Work out the finished part from the listing and answer in its coordinate system (mm). Face numbers are marked on the shaded views. A direction names the side the tool comes from. Coordinates: 2 decimals unless noted, no trailing zeros. Order: outer loops, then holes, each group sorted by start corner. A loop starts at its lowest first (then second) coordinate and runs counter-clockwise, first axis right, second up. Notation, with made-up numbers: M -37,73 L -14,73 A33 cw -14,111 Z; hole C -18.5,85 d11. An arc over 180 degrees is marked long. Use a Markdown table: item, result.
Autodesk Inventor part; units mm, degrees
ref_plane "Work Plane3" through (44.45, 0, 0) normal (-0.342, 0.9397, 0) x (0, 0, -1)
ref_plane "YZ Plane" through (0, 0, 0) normal (1, 0, 0) x (0, 1, 0)
ref_plane "XZ Plane" through (0, 0, 0) normal (0, 1, 0) x (-1, 0, 0)
sketch "Sketch1" plane through (0, 0, 0) normal (0, 1, 0) x (-1, 0, 0)
  line L0 (0, 0) -> (-44.45, 0)
  line L1 (-44.45, 0) -> (-44.45, -25.4)
  line L2 (-44.45, -25.4) -> (0, -25.4)
  line L3 (0, -25.4) -> (0, 0)
  line L4 (-41.275, -25.4) -> (-41.275, 0)
  line L5 (-41.275, -19.05) -> (-44.45, -20.8831)
  line L6 (0, -12.7) -> (-44.45, -12.7) construction
  line L7 (-41.275, -6.35) -> (-44.45, -4.5169)
  point P0 (-44.45, -4.5169)
  point P1 (-41.275, -6.35)
  dimension "d0" = 44.45
  dimension "d7" = 25.4
  dimension "d10" = 3.175
  dimension "d11" = 12.7
  dimension "d12" = 60
extrude "Extrusion1" add sketch "Sketch1" along normal blind 19.05
sketch "Sketch3" plane through (0, 0, 0) normal (0, 0, 1) x (1, 0, 0)
  line L0 (0, 0) -> (44.45, 0)
  line L1 (44.45, 0) -> (44.45, 19.05)
  line L2 (0, 19.05) -> (44.45, 19.05)
  line L3 (0, 0) -> (0, 19.05)
  line L4 (24.8164, 19.05) -> (31.75, 0)
  dimension "d14" = 70
  dimension "d15" = 31.75
sweep "Sweep1" cut profiles "Sketch1" path "Sketch3" path curves L4 contours L4 L7 L1 L0 | L2 L1 L5 L4
ref_plane "Work Plane3" through (44.45, 0, 0) normal (-0.342, 0.9397, 0) x (0, 0, -1)
ref_plane "Work Plane2" through (44.45, 0, 0) normal (-0.9397, -0.342, 0) x (0, 0, -1)
sketch "Sketch5" plane through (44.45, 0, 0) normal (-0.342, 0.9397, 0) x (0, 0, -1)
  point P0 (12.7, 0)
hole "Hole2" at (44.45, 0, -12.7) direction (-0.342, 0.9397, 0) diameter 4.9784 end through all
split "Split1" plane through (44.45, 0, 0) removes the side toward (0.9397, 0.342, 0)
sketch "Sketch4" plane through (0, 19.05, 0) normal (0, 1, 0) x (1, 0, 0)
  line L0 (0, 0) -> (34.3414, 0) construction
  line L1 (0, 25.4) -> (0, 0) construction
  point P0 (17.1707, 12.7)
  point P1 (0, 12.7)
  point P2 (17.1707, 0)
hole "Hole1" at (17.1707, 19.05, -12.7) direction (0, -1, 0) diameter 10.0838 end through all counterbore diameter 15.875 counterbore depth 9.525
equation "\"d14\" = slopeAngle"
equation "\"d18\" = slopeAngle"
equation "\"slopeAngle\" = 70deg"
properties material "Steel, Alloy"
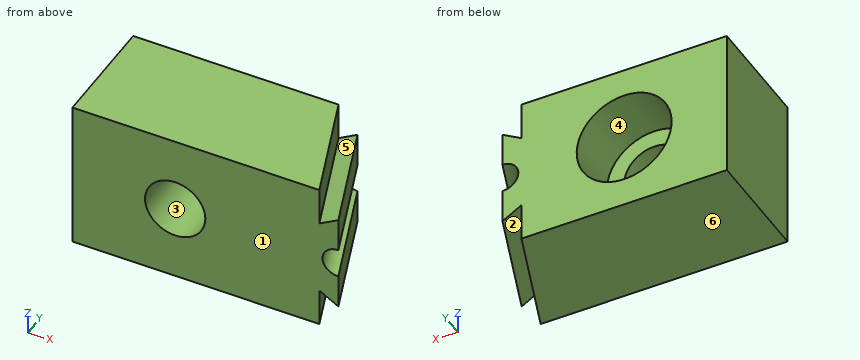
1. For a pull along Z with two mould halves and no side action, classify the marked faces 1, 2 and 3 as +Z half, -Z half, draft (parallel to the pull), parting line (faces both ways), or undercut.
Answers below:
| item | result |
|---|---|
| face 1 | draft |
| face 2 | -Z half |
| face 3 | undercut |
2. Find the intervals of material crossed by probe 1 along Y at (x, z) = (24, -9.75) (3 decimals); probe 2 along X at (y, z) = (16.5, -12.7); probe 3 along Z at (x, y) = (17, 12.75), in increasing order.
Answers below:
| item | result |
|---|---|
| probe 1 | 0 to 9.525 |
| probe 2 | 0 to 9.23, 25.11 to 35.8 |
| probe 3 | -25.4 to -20.64, -4.76 to 0 |
3. For the marked faces 4, 5 and 6, determine the directions among +Z, -Z, +X, -X, +Y, -Y from which every point of the face is accessible in a straight line to the end or side of a thin tool.
Answers below:
| item | result |
|---|---|
| face 4 | +Y |
| face 5 | +Z |
| face 6 | -Z, +X, -X, +Y, -Y |
4. Section A-A on z = -11.5 is taken. Determine the outline of the cut face in (x, y) (3 decimals), then the cut area to 3 significant figures.
Answers below:
| item | result |
|---|---|
| outline | M 0,0 L 12.274,0 L 12.274,9.525 L 9.324,9.525 L 9.324,19.05 L 0,19.05 Z; M 22.068,0 L 42.129,0 L 35.196,19.05 L 25.017,19.05 L 25.017,9.525 L 22.068,9.525 Z |
| area | 494 mm² |
5. Flat-ended cylindrical pins translate along their axes: P1, Ø1.5, axis at y = 16.5, z = -2.5, coming from the -X side; P2, Ø3, axis at y = 2.5, z = -21.5, coming from the +X side; P3, Ø8, axis at x = 20, z = -15, coming from the +Y side (3 decimals); P4, Ø2, axis at x = 37.5, y = 14, coming from the -Z side. Find the tip coordinate at first contact, or state that the pin passes through.
Answers below:
| item | result |
|---|---|
| P1 | x = 0 |
| P2 | x = 44.04 |
| P3 | y = 9.525 |
| P4 | z = -20.43 |
6. Section B-B on x = 10 is taken. Determine the outline of the cut face in (y, z) (3 decimals), then the cut area to 3 significant figures.
Answers below:
| item | result |
|---|---|
| outline | M 0,-25.4 L 19.05,-25.4 L 19.05,-16.104 L 9.525,-16.104 L 9.525,-9.296 L 19.05,-9.296 L 19.05,0 L 0,0 Z |
| area | 419 mm² |
7. Section C-C on z = -5.5 is taken. Determine the outline of the cut face in (x, y) (3 decimals), then the cut area to 3 significant figures.
Answers below:
| item | result |
|---|---|
| outline | M 0,0 L 41.275,0 L 34.341,19.05 L 20.512,19.05 L 20.512,9.525 L 13.829,9.525 L 13.829,19.05 L 0,19.05 Z; M 35.814,19.05 L 42.747,0 L 44.45,0 L 37.516,19.05 Z |
| area | 689 mm² |
8. Section D-D on z = -1.5 is taken. Determine the outline of the cut face in (x, y) (3 decimals).
Answers below:
| item | result |
|---|---|
| outline | M 0,0 L 41.275,0 L 34.341,19.05 L 0,19.05 Z |
